from build123d import *

# Parameters (mm, degrees)
BOSS_EXTRUDE1_DEPTH = 38.1
SKETCH2_R           = 4.4958
CUT_EXTRUDE1_DEPTH  = 25.4
SKETCH4_W           = 14.8336
SKETCH4_H           = 19.9136
BOSS_EXTRUDE2_DEPTH = 37.465


with BuildPart() as part:
    # Sketch1 → Boss-Extrude1 (new body)
    with BuildSketch(Plane(origin=(0, 0, 0), x_dir=(0, 0, -1), z_dir=(1, 0, 0))):
        with BuildLine():
            Line((-6.0706, 6.1341), (-6.0706, -6.1341))
            ThreePointArc((-6.0706, -6.1341), (0, -9.148427884), (6.0706, -6.1341))
            Line((6.0706, -6.1341), (6.0706, 6.1341))
            ThreePointArc((6.0706, 6.1341), (0, 9.148427884), (-6.0706, 6.1341))
        make_face()
    extrude(amount=BOSS_EXTRUDE1_DEPTH)

    # Sketch2 → Cut-Extrude1 (cut)
    with BuildSketch(Plane(origin=(38.1, 0, 0), x_dir=(0, 0, -1), z_dir=(1, 0, 0))):
        Circle(SKETCH2_R)
    extrude(amount=-CUT_EXTRUDE1_DEPTH, mode=Mode.SUBTRACT)

    # Sketch4 → Boss-Extrude2 (add)
    with BuildSketch(Plane.ZY):
        Rectangle(SKETCH4_W, SKETCH4_H)
    extrude(amount=BOSS_EXTRUDE2_DEPTH)


solid = part.part
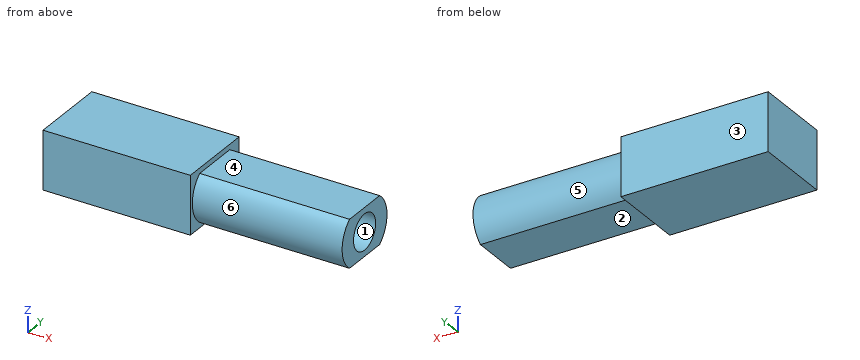
Can you work these out from the model? Positions are in its coordinate system, mm. Face numbers are marked on the shaded views. A direction names the side the tool comes from. Round coordinates to 2 decimals unless told otherwise and drop trailing zeros. Write each loop counter-clockwise with the first axis right and the second up, starting at its lowest first coordinate (ties: lowest second). Pieces come first, ordered by that corner, then holes. Notation, with made-up numbers: (86.25, 41) -> (126.25, 41) arc R25 ccw to (126.25, 67) -> close; hole circle Ø10 at (-15, -23). An arc over 180 degrees is marked (long way). One line per question, with ' | ' between items. Start each with the question number.
1) Suppose I cut it at A-A on x = 20. Write out the boundary of the cut face in (y, z), then the cut area to 3 significant figures.
2) I need wall thicknesses on line 1 (Z direction, x = 10.5, y = 2.75); line 2 (X direction, y = -1.75, z = 6.75) (3 decimals); line 3 (X direction, y = 1.5, z = -1.5) (3 decimals). Which ranges of each line are inside material? Lowest first, please. Write a range as [from, to].
3) If we mould it in two halves opening along Z, with no side actions, what happens to the marked faces 1, 2 and 3? For each: released by +Z, released by -Z, zero draft, split by the parting line, or undercut.
4) I'm going to push flat-ended pins straight in: P1, Ø6, axis at x = 18.5, y = 0.5, coming from the +Z side; P2, Ø6, axis at x = 23.5, z = 4, coming from the -Y side; P3, Ø1, axis at x = 7, z = 2.5, coming from the +Y side. Where does each tip first touch, or does it pass through?
5) Suppose I cut it at C-C on z = 0. Write out the boundary of the cut face in (x, y) (3 decimals).
6) On a 3-axis mill with a long thin cutter (end or side, diameter ignored), from which of +Z, -Z, +X, -X, +Y, -Y can I reach the whole of each face in a straight line? I mean the marked faces 4, 5 and 6. Say none if no direction works.
7) Suppose I cut it at B-B on y = 0. Write out the boundary of the cut face in (x, z) (3 decimals).
Return value:
1) outline: (-6.13, -6.07) -> (6.13, -6.07) arc R7.62 ccw to (6.13, 6.07) -> (-6.13, 6.07) arc R7.62 ccw to start; hole circle Ø8.99 at (0, 0) | area: 137 mm2
2) line 1: z = [-6.07, 6.07] | line 2: x = [-37.465, 0] | line 3: x = [-37.465, 12.7]
3) face 1: undercut | face 2: released by -Z | face 3: zero draft
4) P1: stops at z = 6.07 | P2: stops at y = -9.08 | P3: stops at y = 8.88
5) outline: (-37.465, -9.957) -> (0, -9.957) -> (0, -9.148) -> (38.1, -9.148) -> (38.1, -4.496) -> (12.7, -4.496) -> (12.7, 4.496) -> (38.1, 4.496) -> (38.1, 9.148) -> (0, 9.148) -> (0, 9.957) -> (-37.465, 9.957) -> close
6) face 4: +Z, +X, +Y, -Y | face 5: +X, +Y | face 6: +X, -Y
7) outline: (-37.465, -7.417) -> (0, -7.417) -> (0, -6.071) -> (38.1, -6.071) -> (38.1, -4.496) -> (12.7, -4.496) -> (12.7, 4.496) -> (38.1, 4.496) -> (38.1, 6.071) -> (0, 6.071) -> (0, 7.417) -> (-37.465, 7.417) -> close
